Geometry check sheet. Reference: the model listing, model coordinates, mm. A direction names the side the tool comes from. Round coordinates to 2 decimals unless told otherwise and drop trailing zeros. Loops run counter-clockwise (first coordinate to the right, second up) from the corner with the lowest first, then second, coordinate; pieces in that order, holes last.
```python
from build123d import *

# Parameters (mm, degrees)
SKETCH1_W          = 50.8
SKETCH1_H          = 127
BODY_DEPTH         = 5.334
SKETCH3_W          = 19.05
SKETCH3_H          = 5.334
TOP_TAB_DEPTH      = 5.334
SKETCH4_W          = 19.05
SKETCH4_H          = 5.334
BOT_TAB_DEPTH      = 5.334
SKETCH5_W          = 12.7
SKETCH5_H          = 2.4638
MIDDLE_CUTS_DEPTH  = 74.564469087
SKETCH6_R          = 3.175
BOLTHOLES_DEPTH    = 74.564469087
SKETCH8_W          = 5.334
SKETCH8_H          = 127
PIC_PLATFORM_DEPTH = 95.25
SKETCH10_W         = 19.05
SKETCH10_H         = 5.334
LEFTEXTRUDE_DEPTH  = 5.334
SKETCH11_W         = 19.05
SKETCH11_H         = 5.334
RIGHTEXTRUDE_DEPTH = 5.334


with BuildPart() as part:
    # Sketch1 → body (new body)
    with BuildSketch(Plane.XY):
        Rectangle(SKETCH1_W, SKETCH1_H)
    extrude(amount=BODY_DEPTH)

    # Sketch3 → Top tab (add)
    with BuildSketch(Plane(origin=(0, 63.5, 0), x_dir=(1, 0, 0), z_dir=(0, 1, 0))):
        with Locations((0, -2.667)):
            Rectangle(SKETCH3_W, SKETCH3_H)
    extrude(amount=TOP_TAB_DEPTH)

    # Sketch4 → Bot tab (add)
    with BuildSketch(Plane.XZ.offset(63.5)):
        with Locations((0, 2.667)):
            Rectangle(SKETCH4_W, SKETCH4_H)
    extrude(amount=BOT_TAB_DEPTH)

    # Sketch5 → middle cuts (cut, through all)
    with BuildSketch(Plane.XY.offset(5.334)):
        with Locations((-13.649999878, 24.909253458)):
            Rectangle(SKETCH5_W, SKETCH5_H)
        with Locations((13.649999878, -28.354546542)):
            Rectangle(SKETCH5_W, SKETCH5_H)
        with Locations((-13.649999878, -28.354546542)):
            Rectangle(SKETCH5_W, SKETCH5_H)
        with Locations((13.649999878, 24.909253458)):
            Rectangle(SKETCH5_W, SKETCH5_H)
    extrude(amount=-MIDDLE_CUTS_DEPTH, mode=Mode.SUBTRACT)

    # Sketch6 → BoltHoles (cut, through all)
    with BuildSketch(Plane.XY.offset(5.334)):
        with Locations((13.900024524, 50.8)):
            Circle(SKETCH6_R)
        with Locations((13.900024524, -50.8)):
            Circle(SKETCH6_R)
    extrude(amount=-BOLTHOLES_DEPTH, mode=Mode.SUBTRACT)

    # Sketch8 → PIC platform (add)
    with BuildSketch(Plane.ZY.offset(25.4)):
        with Locations((2.667, 0)):
            Rectangle(SKETCH8_W, SKETCH8_H)
    extrude(amount=PIC_PLATFORM_DEPTH)

    # Sketch10 → LeftExtrude (add)
    with BuildSketch(Plane(origin=(0, 63.5, 0), x_dir=(1, 0, 0), z_dir=(0, 1, 0))):
        with Locations((-98.425, -2.667)):
            Rectangle(SKETCH10_W, SKETCH10_H)
    extrude(amount=LEFTEXTRUDE_DEPTH)

    # Sketch11 → RightExtrude (add)
    with BuildSketch(Plane.XZ.offset(63.5)):
        with Locations((-98.425, 2.667)):
            Rectangle(SKETCH11_W, SKETCH11_H)
    extrude(amount=RIGHTEXTRUDE_DEPTH)


solid = part.part
```
1) Sectioned sample at B-B, the plane y = -50.8. Record the cut outline in (x, z).
Report:
outline: (-120.65, 0) - (10.73, 0) - (10.73, 5.33) - (-120.65, 5.33) - close; (17.08, 0) - (25.4, 0) - (25.4, 5.33) - (17.08, 5.33) - close
2) Gauge pin test, flat ends, axial feed: pin 1 (1.6 mm diameter, centred on x = 14.5, z = 2.5, fed in from +Y); pin 2 (2.5 mm diameter, centred on y = 66.5, z = 3.5, fed in from +X) (3 decimals); pin 3 (1 mm diameter, centred on x = -49.5, z = 4, fed in from -Y). Record the tip position at first contact, or that the pin passes through.
Report:
pin 1: stops at y = 63.5
pin 2: stops at x = 9.525
pin 3: stops at y = -63.5
3) Mould release check, pull along Y, two halves, no side actions. Record for faces 4 (the face through (-9.525, -66, 3)), 5 (the face through (-49, -63.5, 3)), 6 (the face through (14, -29.586, 3)): +Y half, -Y half, draft (parallel to the pull), parting line (faces both ways), or undercut.
Report:
face 4: draft
face 5: -Y half
face 6: undercut
4) Sectioned sample at C-C, the plane z = 2.05. State how many separate pieces and enclosed holes the cut face has, then the cut area to 3 significant figures.
Report:
separate pieces: 1
enclosed holes: 6
area: 18,800 mm2
5) Access from +Z, -Z, +X, -X, +Y, -Y to the whole of each face (thin tool, end or side, straight path). Record for faces 1 (the face through (-14, -29.586, 3)), 2 (the face through (-88.9, 66, 3)), 3 (the face through (-107.95, -66, 3)).
Report:
face 1: +Z, -Z
face 2: +Z, -Z, +Y
face 3: +Z, -Z, -X, -Y
6) Sectioned sample at A-A, the plane x = -17. Record the cut outline in (y, z), then the cut area to 3 significant figures.
Report:
outline: (-63.5, 0) - (-29.59, 0) - (-29.59, 5.33) - (-63.5, 5.33) - close; (-27.12, 0) - (23.68, 0) - (23.68, 5.33) - (-27.12, 5.33) - close; (26.14, 0) - (63.5, 0) - (63.5, 5.33) - (26.14, 5.33) - close
area: 651 mm2
7) Scan lines: line 1 along Y through (x, z) = (-10, 1.3); line 2 along Y through (x, z) = (-51, 1.9). Record each from-to range of solid material in increasing order.
Report:
line 1: y = -63.5 to -29.59, -27.12 to 23.68, 26.14 to 63.5
line 2: y = -63.5 to 63.5
